Check sheet for the modelled part. Datum: model origin and axes. Units: mm. Face numbers are marked on the shaded views. A direction names the side the tool comes from. Round coordinates to 2 decimals unless told otherwise and drop trailing zeros. Loops run counter-clockwise (first coordinate to the right, second up) from the corner with the lowest first, then second, coordinate; pieces in that order, holes last. Notation, with made-up numbers: M 85,8.5 L 92,8.5 A29 cw 92,31.5 Z; hole C 57.25,27 d2. An arc over 180 degrees is marked long. One line per question, with ' | ' between items. Start each with the question number.
(1) Section check C-C (z = -3.25). Record the boundary of the cut face in (x, y).
(2) Thickness scan on probe 1 along X at (y, z) = (11.5, 7.25); probe 2 along Y at (x, z) = (7.5, 0); probe 3 along Z at (x, y) = (-14, 11). Record the ranges inside material, lowest first. Write a range as [from, to].
(3) Go/stop test with flat-tipped pins: P1, Ø2, axis at x = 18, y = 5.5, coming from the +Z side; P2, Ø4, axis at x = 7.5, y = 8.5, coming from the -Z side; P3, Ø2, axis at y = 8.5, z = 4.5, coming from the -X side. Record where each tip stops, or that it passes through.
(4) Tool access check on the marked faces 4, 5, 6 and 7. Record the directions out of +Z, -Z, +X, -X, +Y, -Y that give a thin tool (end or side, any length) a straight path to the whole face; none if there is none.
(5) Section check B-B (y = 1.5). Record the boundary of the cut face in (x, z) (3 decimals).
(6) Section check D-D (x = -14). Record the boundary of the cut face in (y, z), and give its area (4 significant figures).
(7) Section check A-A (x = -4.75). Record the boundary of the cut face in (y, z) (3 decimals), and give its area (3 significant figures).
(8) Draft check along Z on the marked faces 1, 2 and 3. Enter one of: +Z half, -Z half, draft (parallel to the pull), parting line (faces both ways), or undercut.
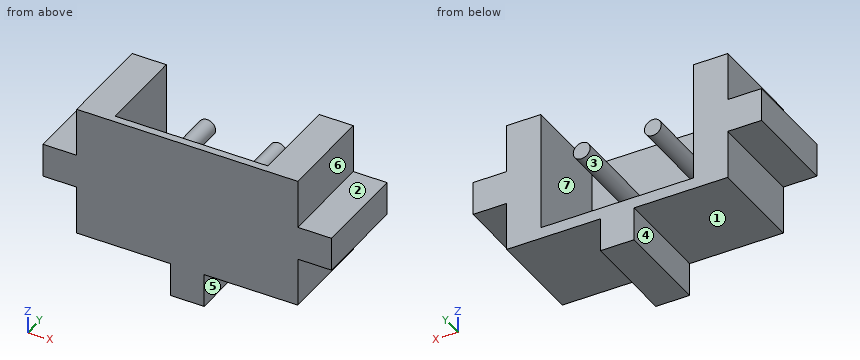
```python
from build123d import *

# Parameters (mm, degrees)
SALIENTE_EXTRUIR1_DEPTH = 13
CROQUIS4_W              = 20.4
CROQUIS4_H              = 16
CROQUIS4_R              = 1.125
CORTAR_EXTRUIR1_DEPTH   = 12


with BuildPart() as part:
    # Croquis2 → Saliente-Extruir1 (new body)
    with BuildSketch(Plane(origin=(0, 0, 0), x_dir=(1, 0, 0), z_dir=(0, 1, 0))):
        Polygon((14.75, -8.75), (-14.75, -8.75), (-14.75, -2.25), (-19.25, -2.25), (-19.25, 2.25), (-14.75, 2.25), (-14.75, 8.75), (-2.25, 8.75), (-2.25, 13.25), (2.25, 13.25), (2.25, 8.75), (14.75, 8.75), (14.75, 2.25), (19.25, 2.25), (19.25, -2.25), (14.75, -2.25), align=None)
    extrude(amount=SALIENTE_EXTRUIR1_DEPTH)

    # Croquis4 → Cortar-Extruir1 (cut)
    with BuildSketch(Plane(origin=(0, 13, 0), x_dir=(1, 0, 0), z_dir=(0, 1, 0))):
        with Locations((0, -0.75)):
            Rectangle(CROQUIS4_W, CROQUIS4_H)
        with Locations(Location((4.75, -1.75, 0), (0, 0, 270))):
            Circle(CROQUIS4_R, mode=Mode.SUBTRACT)
        with Locations(Location((-4.75, -1.75, 0), (0, 0, 270))):
            Circle(CROQUIS4_R, mode=Mode.SUBTRACT)
    extrude(amount=-CORTAR_EXTRUIR1_DEPTH, mode=Mode.SUBTRACT)


solid = part.part
```
The answers:
1) outline: M -14.75,0 L 14.75,0 L 14.75,13 L 10.2,13 L 10.2,1 L -10.2,1 L -10.2,13 L -14.75,13 Z
2) probe 1: [-14.75, -10.2], [10.2, 14.75] | probe 2: [0, 1] | probe 3: [-8.75, 8.75]
3) P1: z = 2.25 | P2: z = -8.75 | P3: x = -14.75
4) face 4: -Z, -X, +Y, -Y | face 5: -Z, +X, +Y, -Y | face 6: +Z, +X, +Y, -Y | face 7: +Z, +Y
5) outline: M -19.25,-2.25 L -14.75,-2.25 L -14.75,-8.75 L -2.25,-8.75 L -2.25,-13.25 L 2.25,-13.25 L 2.25,-8.75 L 14.75,-8.75 L 14.75,-2.25 L 19.25,-2.25 L 19.25,2.25 L 14.75,2.25 L 14.75,8.75 L 10.2,8.75 L 10.2,-7.25 L -10.2,-7.25 L -10.2,8.75 L -14.75,8.75 L -14.75,2.25 L -19.25,2.25 Z; C -4.75,1.75 d2.25; C 4.75,1.75 d2.25
6) outline: M 0,-8.75 L 13,-8.75 L 13,8.75 L 0,8.75 Z | area: 227.5 mm²
7) outline: M 0,-8.75 L 13,-8.75 L 13,-7.25 L 1,-7.25 L 1,0.625 L 13,0.625 L 13,2.875 L 1,2.875 L 1,8.75 L 0,8.75 Z | area: 62.5 mm²
8) face 1: -Z half | face 2: +Z half | face 3: undercut
